Read the model definition and answer for the solid it produces. Units are mm, in the model's axes. Face numbers are marked on the shaded views. A direction names the side the tool comes from. Round coordinates to 2 decimals unless told otherwise and drop trailing zeros. Write each loop counter-clockwise with the first axis right and the second up, starting at its lowest first coordinate (ties: lowest second). Pieces come first, ordered by that corner, then holes. Notation, with made-up numbers: (-25.75, 29.25) - (6.25, 29.25) arc R8 cw to (6.25, 42.25) - close; hole circle Ø7 at (16.25, 1.5). An arc over 180 degrees is marked (long way). Use one line per item in the form item = value. Start each with the question number.
1) Consider line 1 along Z through (x, y) = (-3.25, 6.5); line 2 along Z through (x, y) = (7.5, 3.25); line 3 along Y through (x, z) = (2.5, 4.5). Determine where each line is inside the solid, lowest interval first. Write a range as from..to.
2) The part is cut by section C-C, the plane z = 11. Give the vertices of the cut face in (x, y), plus the area to 3 significant figures.
3) The part is cut by section A-A, the plane y = 0. Give the vertices of the cut face in (x, z), plus the area to 3 significant figures.
4) For the marked faces 1 and 2, determine the directions among +Z, -Z, +X, -X, +Y, -Y from which every point of the face is accessible in a straight line to the end or side of a thin tool.
5) Each of these flat-tipped pins is pushed along its axis until it touches: pin 1 (1.5 mm diameter, centred on y = -2.5, z = 13.5, fed in from +X); pin 2 (1.5 mm diameter, centred on x = -5, z = 16.5, fed in from -Y); pin 3 (2 mm diameter, centred on y = -6.5, z = 10.5, fed in from -X). Where does it stop, or does it pass through?
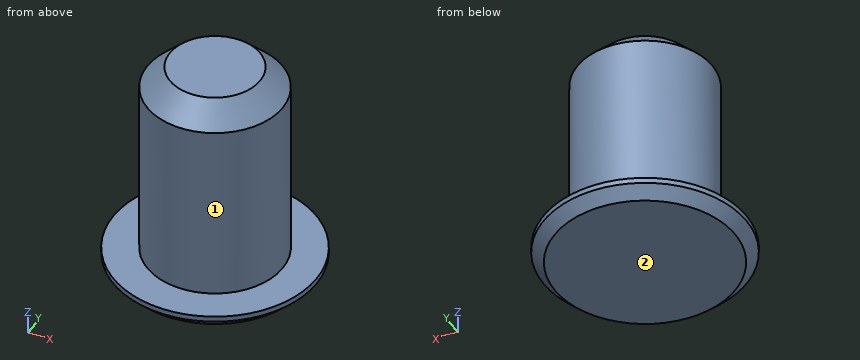
from build123d import *

# Parameters (mm, degrees)
SKETCH_R        = 9
PAD_DEPTH       = 1.5
SKETCH001_R     = 6
PAD001_DEPTH    = 18
CHAMFER_SIZE    = 1
CHAMFER001_SIZE = 2


with BuildPart() as part:
    # Sketch → Pad (new body)
    with BuildSketch(Plane.XY):
        Circle(SKETCH_R)
    extrude(amount=PAD_DEPTH)

    # Sketch001 (on Face3 of Pad) → Pad001 (join)
    with BuildSketch(Plane.XY.offset(1.5)):
        Circle(SKETCH001_R)
    extrude(amount=PAD001_DEPTH)

    # Chamfer
    chamfer_edges = [part.edges().sort_by_distance(p)[0] for p in [
        (-9, 0, 0),
    ]]
    chamfer(chamfer_edges, length=CHAMFER_SIZE)

    # Chamfer001
    chamfer001_edges = [part.edges().sort_by_distance(p)[0] for p in [
        (-6, 0, 19.5),
    ]]
    chamfer(chamfer001_edges, length=CHAMFER001_SIZE)


solid = part.part
Geometry results:
q1.line_1 = 0..1.5
q1.line_2 = 0.17..1.5
q1.line_3 = -5.45..5.45
q2.outline = circle Ø12 at (0, 0)
q2.area = 113 mm2
q3.outline = (-9, 1) - (-8, 0) - (8, 0) - (9, 1) - (9, 1.5) - (6, 1.5) - (6, 17.5) - (4, 19.5) - (-4, 19.5) - (-6, 17.5) - (-6, 1.5) - (-9, 1.5) - close
q3.area = 238 mm2
q4.face_1 = +Z
q4.face_2 = -Z, +X, -X, +Y, -Y
q5.pin_1 = 5.74
q5.pin_2 = -4.24
q5.pin_3 = -2.4
